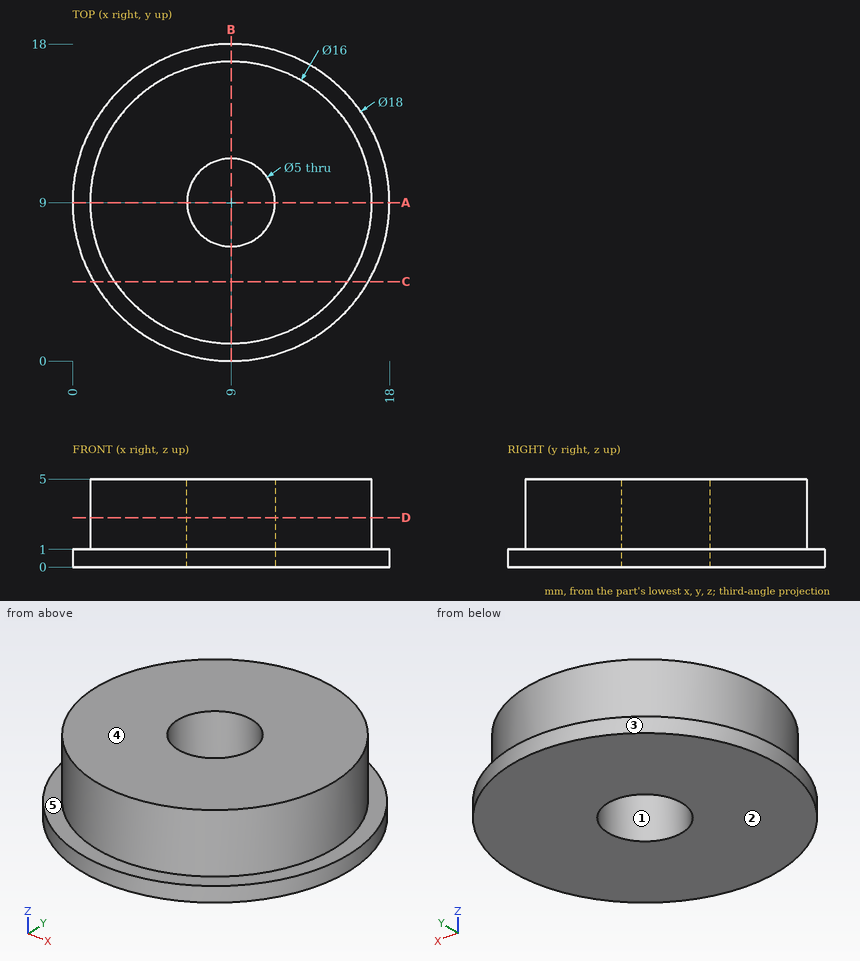
Verification items for this drawing (mm, ordinates from the low corner). A direction names the side the tool comes from. Round coordinates to 2 decimals unless told otherwise and drop trailing zeros. Write each loop counter-clockwise with the first axis right and the second up, starting at its lowest first coordinate (ties: lowest second). Pieces come first, ordered by that corner, then holes. Notation, with made-up numbers: M 65,33.25 L 80,33.25 A12 cw 80,37.25 Z; hole C -19,-23 d8. An arc over 180 degrees is marked long. Write item = value, one per line. Start each with the question number.
1. Gauge pin test, flat end, axial feed: pin 1 (1.5 mm diameter, centred on y = 12, z = 2.5, fed in from -X). Record the tip position at first contact, or that the pin passes through.
2. Section check A-A, the plane y = 9. Record the cut outline in (x, z).
3. Scan lines: line 1 (Y direction, x = 9, z = 2.25); line 2 (X direction, y = 2.75, z = 1.55); line 3 (Z direction, x = 7.75, y = 1). Record each from-to range of solid material in increasing order. Write a range as [from, to].
4. Section check C-C, the plane y = 4.5. Record the cut outline in (x, z).
5. Release check for a two-part mould opening along X. For the marked faces 1, 2 and 3 record: pulls with the +X half, pulls with the -X half, needs draft (parallel to the pull), parting line crosses it, or undercut.
6. Section check D-D, the plane z = 2.8. Record the cut outline in (x, y), then the cut area to 3 significant figures.
7. Tool access check on the marked faces 4 and 5. Record the directions out of +Z, -Z, +X, -X, +Y, -Y that give a thin tool (end or side, any length) a straight path to the whole face; none if there is none.
Results found:
q1.pin_1 = 1.32
q2.outline = M 0,0 L 6.5,0 L 6.5,5 L 1,5 L 1,1 L 0,1 Z; M 11.5,0 L 18,0 L 18,1 L 17,1 L 17,5 L 11.5,5 Z
q3.line_1 = [1, 6.5], [11.5, 17]
q3.line_2 = [4.01, 13.99]
q3.line_3 = [0, 1]
q4.outline = M 1.21,0 L 16.79,0 L 16.79,1 L 15.61,1 L 15.61,5 L 2.39,5 L 2.39,1 L 1.21,1 Z
q5.face_1 = undercut
q5.face_2 = needs draft
q5.face_3 = parting line crosses it
q6.outline = C 9,9 d16; hole C 9,9 d5
q6.area = 181 mm^2
q7.face_4 = +Z, +X, -X, +Y, -Y
q7.face_5 = +Z
